Autodesk Inventor part; units mm, degrees
ref_plane "YZ Plane" through (0, 0, 0) normal (1, 0, 0) x (0, 1, 0)
ref_plane "XZ Plane" through (0, 0, 0) normal (0, 1, 0) x (-1, 0, 0)
ref_plane "XY Plane" through (0, 0, 0) normal (0, 0, 1) x (1, 0, 0)
sketch "Sketch1" plane through (0, 0, 0) normal (0, 0, 1) x (1, 0, 0)
  line L0 (0, 0) -> (40, 0)
  line L1 (40, 0) -> (40, 20)
  line L2 (40, 20) -> (0, 20)
  line L3 (0, 20) -> (0, 0)
extrude "Extrusion1" add sketch "Sketch1" along normal blind 10
sketch "Sketch2" plane through (0, 0, 0) normal (0, 0, 1) x (1, 0, 0)
  line L0 (10, 5) -> (30, 5)
  line L1 (30, 5) -> (30, 15)
  line L2 (30, 15) -> (10, 15)
  line L3 (10, 15) -> (10, 5)
extrude "Extrusion2" cut sketch "Sketch2" along normal blind 5
properties part number "17_box_cut"
Here's how the part is built. I have some questions about the finished solid (model axes, mm). A direction names the side the tool comes from. Round coordinates to 2 decimals unless told otherwise and drop trailing zeros. Order: outer loops, then holes, each group sorted by start corner. A loop starts at its lowest first (then second) coordinate and runs counter-clockwise, first axis right, second up. Notation, with made-up numbers: (61, 21.5) -> (71, 21.5) arc R13 ccw to (71, 28.5) -> close; hole circle Ø2 at (83.25, 32). An arc over 180 degrees is marked (long way). Use a Markdown table: item, result. Add a question column.
(1) Suppose I cut it at A-A, the plane y = 8.75. Please give me the cut outline in (x, z), and give its area (3 significant figures).
(2) If we mould it in two halves opening along X, with no side actions, what happens to faces 1 (the face through (20, 17, 0)), 2 (the face through (20, 10, 5)), 3 (the face through (0, 10, 5)), 4 (the face through (10, 10, 2))? For each: released by +X, released by -X, zero draft, split by the parting line, or undercut.
(3) I need wall thicknesses on line 1 along Y through (x, z) = (23.5, 4.5); line 2 along X through (y, z) = (13, 4.5); line 3 along Z through (x, y) = (20.5, 13.25). Which ranges of each line are inside material? Lowest first, please.
(4) Suppose I cut it at B-B, the plane z = 1.75. Please give me the cut outline in (x, y).
(5) For pin 1 Ø1.5 at (y, z) = (15.5, 1) entering from -X; pin 2 Ø3 at (x, y) = (20, 9) entering from -Z, each with a flat end and sliding along its axis, tell me the tip position at first contact or that it passes through.
(6) Suppose I cut it at C-C, the plane x = 28. Please give me the cut outline in (y, z).
(7) For faces 5 (the face through (20, 15, 2)), 6 (the face through (40, 10, 5)), which set-ups out of +Z, -Z, +X, -X, +Y, -Y let a thin tool reach every point of the face, with its end or its side?
Verdict:
| question | item | result |
|---|---|---|
| 1 | outline | (0, 0) -> (10, 0) -> (10, 5) -> (30, 5) -> (30, 0) -> (40, 0) -> (40, 10) -> (0, 10) -> close |
| 1 | area | 300 mm2 |
| 2 | face 1 | zero draft |
| 2 | face 2 | undercut |
| 2 | face 3 | released by -X |
| 2 | face 4 | undercut |
| 3 | line 1 | 0 to 5, 15 to 20 |
| 3 | line 2 | 0 to 10, 30 to 40 |
| 3 | line 3 | 5 to 10 |
| 4 | outline | (0, 0) -> (40, 0) -> (40, 20) -> (0, 20) -> close; hole (10, 5) -> (30, 5) -> (30, 15) -> (10, 15) -> close |
| 5 | pin 1 | x = 0 |
| 5 | pin 2 | z = 5 |
| 6 | outline | (0, 0) -> (5, 0) -> (5, 5) -> (15, 5) -> (15, 0) -> (20, 0) -> (20, 10) -> (0, 10) -> close |
| 7 | face 5 | -Z |
| 7 | face 6 | +Z, -Z, +X, +Y, -Y |
